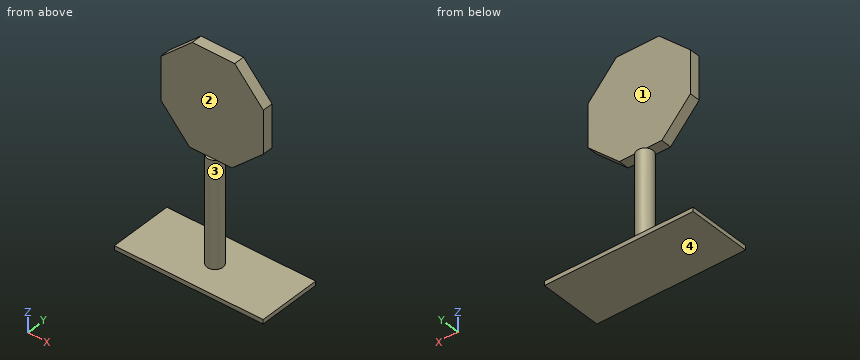
Autodesk Inventor part; units mm, degrees
ref_plane "YZ Plane" through (0, 0, 0) normal (1, 0, 0) x (0, 1, 0)
ref_plane "XZ Plane" through (0, 0, 0) normal (0, 1, 0) x (-1, 0, 0)
ref_plane "XY Plane" through (0, 0, 0) normal (0, 0, 1) x (1, 0, 0)
sketch "Skizze1" plane through (0, 0, 0) normal (0, 1, 0) x (-1, 0, 0)
  line L0 (35.5112, -88.3128) -> (35.5112, -108.3128)
  line L1 (35.5112, -108.3128) -> (22.0645, -123.1178)
  line L2 (22.0645, -123.1178) -> (2.0645, -123.1178)
  line L3 (2.0645, -123.1178) -> (-12.7404, -109.6711)
  line L4 (-12.7404, -109.6711) -> (-12.7404, -89.6711)
  line L5 (-12.7404, -89.6711) -> (0.7063, -74.8661)
  line L6 (0.7063, -74.8661) -> (20.7063, -74.8661)
  line L7 (20.7063, -74.8661) -> (35.5112, -88.3128)
  point P0 (0, 0)
  dimension "d0" = 20
  dimension "d1" = 20
  dimension "d2" = 20
  dimension "d3" = 20
  dimension "d4" = 20
  dimension "d5" = 20
  dimension "d6" = 20
  dimension "d7" = 20
extrude "Extrusion1" add sketch "Skizze1" along normal blind 5
sketch "Skizze2" plane through (-2.0645, 0, -123.1178) normal (0, 0, -1) x (-1, 0, 0)
  circle A0 centre (10, 2.5) radius 3.75
  line L0 (0, 5) -> (20, 5)
  point P0 (-2.0645, 0)
  dimension "d11" = 7.5
  dimension "d12" = 2.5
extrude "Extrusion2" add sketch "Skizze2" along normal blind 51.748
sketch "Skizze3" plane through (-12.0645, 2.5, -174.8658) normal (0, 0, -1) x (-1, 0, 0)
  line L0 (-35, -15) -> (35, -15)
  line L1 (35, -15) -> (35, 15)
  line L2 (35, 15) -> (-35, 15)
  line L3 (-35, 15) -> (-35, -15)
  arc A0 (-2.7951, 2.5) -> (-2.7951, -2.5) centre (0, 0) ccw
  line L4 (-35, -15) -> (35, 15) construction
  line L5 (35, -15) -> (-35, 15) construction
  point P0 (-12.0645, -2.5)
  dimension "d15" = 70
  dimension "d16" = 30
extrude "Extrusion3" add sketch "Skizze3" against normal blind 2
sketch "Skizze4" plane through (0, 5, 0) normal (0, 1, 0) x (1, 0, 0)
  point P0 (0, 0)
properties part number "Stoppschild_klein 10 cm Höhe"
Input: part model. Units: mm. Frame: model coordinates. Face numbers are marked on the shaded views. A direction names the side the tool comes from. Coordinates: 2 decimals unless noted, no trailing zeros. Write each loop counter-clockwise with the first axis right and the second up, starting at its lowest first coordinate (ties: lowest second). Pieces come first, ordered by that corner, then holes. Notation, with made-up numbers: (60, 10.5) -> (74, 10.5) arc R21 cw to (74, 40.5) -> close; hole circle Ø2 at (40.5, -10.75). An arc over 180 degrees is marked (long way). Write each question's results on one line, items separated by ' | '.
Item 1: Pin query (flat end, axial travel): pin 1 Ø4 at (y, z) = (2.5, -104.5) entering from +X; pin 2 Ø6 at (x, y) = (-5.5, -3.5) entering from +Z; pin 3 Ø3 at (x, z) = (-9, -93) entering from +Y. Return the tip coordinate at first contact, or that it passes through.
Conclusion:
pin 1: stops at x = 12.74 | pin 2: stops at z = -172.87 | pin 3: stops at y = 5
Item 2: Section query C-C on z = -91.5. Return loops of the section in (x, y), plus the area to 3 significant figures.
Conclusion:
outline: (-35.51, 0) -> (12.74, 0) -> (12.74, 5) -> (-35.51, 5) -> close | area: 241 mm^2
Item 3: Section query B-B on y = 2.5. Return loops of the section in (x, z).
Conclusion:
outline: (-47.06, -174.87) -> (22.94, -174.87) -> (22.94, -172.87) -> (-8.31, -172.87) -> (-8.31, -123.12) -> (-2.06, -123.12) -> (12.74, -109.67) -> (12.74, -89.67) -> (-0.71, -74.87) -> (-20.71, -74.87) -> (-35.51, -88.31) -> (-35.51, -108.31) -> (-22.06, -123.12) -> (-15.81, -123.12) -> (-15.81, -172.87) -> (-47.06, -172.87) -> close
Item 4: Material intervals for probe 1 along Z at (x, y) = (-28.5, -8); probe 2 along Y at (x, z) = (7, -98); probe 3 along Z at (x, y) = (-31, 1.75), sorted ascending.
Conclusion:
probe 1: z = -174.87 to -172.87 | probe 2: y = 0 to 5 | probe 3: z = -174.87 to -172.87, -113.28 to -84.22
Item 5: Section query A-A on x = -32.5. Return loops of the section in (y, z), plus the area to 3 significant figures.
Conclusion:
outline: (-12.5, -174.87) -> (17.5, -174.87) -> (17.5, -172.87) -> (-12.5, -172.87) -> close; (0, -111.63) -> (5, -111.63) -> (5, -85.58) -> (0, -85.58) -> close | area: 190 mm^2
Item 6: Set-up query: the marked faces 1, 2, 3 and 4. Return all of +Z, -Z, +X, -X, +Y, -Y with unobstructed straight access to the full face (end or side cutting, diameter ignored); none if empty.
Conclusion:
face 1: +Z, +X, -X, +Y | face 2: +Z, +X, -X, -Y | face 3: none | face 4: -Z, +X, -X, +Y, -Y
Item 7: Section query D-D on x = -39.5. Return loops of the section in (y, z).
Conclusion:
outline: (-12.5, -174.87) -> (17.5, -174.87) -> (17.5, -172.87) -> (-12.5, -172.87) -> close
